Check sheet for the drawn part. Datum: minimum x, y, z corner. Units: mm. A direction names the side the tool comes from. Coordinates: 2 decimals unless noted, no trailing zeros. Write each loop counter-clockwise with the first axis right and the second up, starting at its lowest first coordinate (ties: lowest second). Pieces come first, ordered by that corner, then holes. Notation, with made-up numbers: (76.25, 54) -> (99.25, 54) arc R11 cw to (99.25, 73) -> close; hole circle Ø9 at (-36.5, 67). An arc over 180 degrees is marked (long way). Write item = value, one per line. Start each with the question number.
(1) Section check B-B (x = 9.5). Record the cut outline in (y, z), plus the area to 3 significant figures.
(2) Section check A-A (y = 2.25). Record the cut outline in (x, z).
(3) Gauge pin test, flat ends, axial feed: pin 1 Ø1 at (y, z) = (15, 2) entering from +X; pin 2 Ø1.2 at (x, z) = (9, 2.5) entering from -Y; pin 3 Ø1 at (x, z) = (2.5, 1.5) entering from +Y; pin 4 Ø3 at (x, y) = (12.5, 2.5) entering from -Z. Record the tip position at first contact, or that the pin passes through.
(4) Set-up check for the marked faces 1, 2 and 3: record each of +Z, -Z, +X, -X, +Y, -Y from which the full face is reachable in a straight line by a thin tool's end or side.
(5) Section check D-D (x = 15.5). Record the cut outline in (y, z), plus the area to 3 significant figures.
(6) Material ranges on probe 1 along X at (y, z) = (1, 1.95); probe 2 along Y at (x, z) = (8.25, 2.4); probe 3 along X at (y, z) = (10, 1.8), recorded low to high. Write a range as [from, to].
(7) Section check C-C (z = 1.5). Record the cut outline in (x, y), plus the area to 3 significant figures.
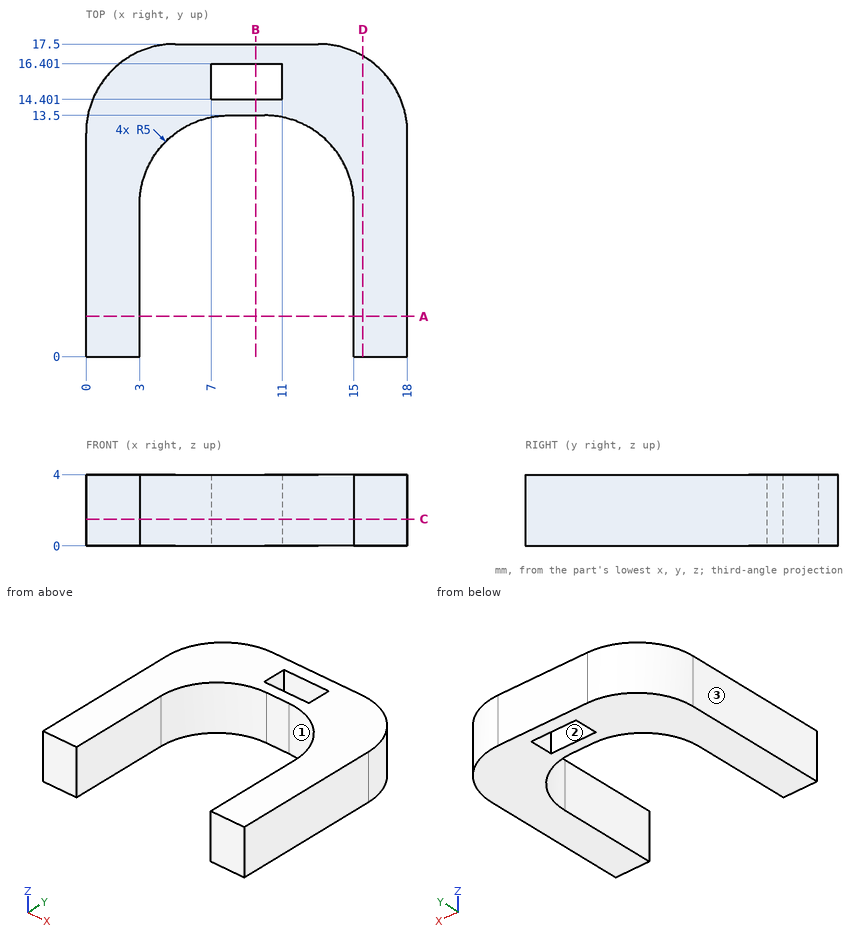
Response:
q1.outline = (13.5, 0) -> (14.4, 0) -> (14.4, 4) -> (13.5, 4) -> close; (16.4, 0) -> (17.5, 0) -> (17.5, 4) -> (16.4, 4) -> close
q1.area = 8.00 mm2
q2.outline = (0, 0) -> (3, 0) -> (3, 4) -> (0, 4) -> close; (15, 0) -> (18, 0) -> (18, 4) -> (15, 4) -> close
q3.pin_1 = 17.58
q3.pin_2 = 13.5
q3.pin_3 = 17.08
q3.pin_4 = through
q4.face_1 = +Z, -Z, -Y
q4.face_2 = +Z, -Z
q4.face_3 = +Z, -Z, -X, +Y, -Y
q5.outline = (0, 0) -> (16.83, 0) -> (16.83, 4) -> (0, 4) -> close
q5.area = 67.3 mm2
q6.probe_1 = [0, 3], [15, 18]
q6.probe_2 = [13.5, 14.4], [16.4, 17.5]
q6.probe_3 = [0, 3.23], [14.77, 18]
q7.outline = (0, 0) -> (3, 0) -> (3, 8.5) arc R5 cw to (8, 13.5) -> (10, 13.5) arc R5 cw to (15, 8.5) -> (15, 0) -> (18, 0) -> (18, 12.5) arc R5 ccw to (13, 17.5) -> (5, 17.5) arc R5 ccw to (0, 12.5) -> close; hole (7, 14.4) -> (11, 14.4) -> (11, 16.4) -> (7, 16.4) -> close
q7.area = 145 mm2
